Autodesk Inventor part; units mm, degrees
ref_plane "YZ Plane" through (0, 0, 0) normal (1, 0, 0) x (0, 1, 0)
ref_plane "XZ Plane" through (0, 0, 0) normal (0, 1, 0) x (-1, 0, 0)
ref_plane "XY Plane" through (0, 0, 0) normal (0, 0, 1) x (1, 0, 0)
sketch "Sketch2" plane through (0, 0, 0) normal (0, 0, 1) x (0, 1, 0)
  line L0 (24.9, -57.75) -> (24.9, -91.85)
  circle A0 centre (24.9, -74.8) radius 17.05
  circle A1 centre (24.9, -74.8) radius 0.9375
  line L1 (24.9, -74.8) -> (36.9562, -86.8562)
  line L2 (24.9, -74.8) -> (41.95, -74.8) construction
  line L3 (26.7738, -76.6738) -> (35.0823, -84.9823) construction
  line L4 (26.3319, -77.1158) -> (34.6404, -85.4243)
  line L5 (35.5243, -84.5404) -> (27.2158, -76.2319)
  arc A2 (27.2158, -76.2319) -> (26.3319, -77.1158) centre (26.7738, -76.6738) ccw
  arc A3 (34.6404, -85.4243) -> (35.5243, -84.5404) centre (35.0823, -84.9823) ccw
  line L6 (30.9281, -80.8281) -> (42.6781, -80.8281) construction
  line L7 (34.8, -54.9) -> (34.8, -60.9186) construction
  line L8 (32.3, -54.9) -> (32.3, -60.9186)
  line L9 (37.3, -60.9186) -> (37.3, -54.9)
  arc A4 (37.3, -54.9) -> (32.3, -54.9) centre (34.8, -54.9) ccw
  arc A5 (32.3, -60.9186) -> (37.3, -60.9186) centre (34.8, -60.9186) ccw
  line L10 (15, -54.9) -> (15, -60.9186) construction
  line L11 (12.5, -54.9) -> (12.5, -60.9186)
  line L12 (17.5, -60.9186) -> (17.5, -54.9)
  arc A6 (17.5, -54.9) -> (12.5, -54.9) centre (15, -54.9) ccw
  arc A7 (12.5, -60.9186) -> (17.5, -60.9186) centre (15, -60.9186) ccw
  line L13 (15, -94.7) -> (15, -88.6814) construction
  line L14 (17.5, -94.7) -> (17.5, -88.6814)
  line L15 (12.5, -88.6814) -> (12.5, -94.7)
  arc A8 (12.5, -94.7) -> (17.5, -94.7) centre (15, -94.7) ccw
  arc A9 (17.5, -88.6814) -> (12.5, -88.6814) centre (15, -88.6814) ccw
  line L16 (34.8, -94.7) -> (34.8, -88.6814) construction
  line L17 (37.3, -94.7) -> (37.3, -88.6814)
  line L18 (32.3, -88.6814) -> (32.3, -94.7)
  arc A10 (32.3, -94.7) -> (37.3, -94.7) centre (34.8, -94.7) ccw
  arc A11 (37.3, -88.6814) -> (32.3, -88.6814) centre (34.8, -88.6814) ccw
  line L19 (39.3, -74.175) -> (27.55, -74.175)
  arc A12 (39.3, -75.425) -> (39.3, -74.175) centre (39.3, -74.8) ccw
  line L20 (27.55, -75.425) -> (39.3, -75.425)
  arc A13 (27.55, -74.175) -> (27.55, -75.425) centre (27.55, -74.8) ccw
  line L21 (34.6404, -64.1757) -> (26.3319, -72.4842)
  arc A14 (35.5243, -65.0596) -> (34.6404, -64.1757) centre (35.0823, -64.6177) ccw
  line L22 (27.2158, -73.3681) -> (35.5243, -65.0596)
  arc A15 (26.3319, -72.4842) -> (27.2158, -73.3681) centre (26.7738, -72.9262) ccw
  line L23 (24.275, -60.4) -> (24.275, -72.15)
  arc A16 (25.525, -60.4) -> (24.275, -60.4) centre (24.9, -60.4) ccw
  line L24 (25.525, -72.15) -> (25.525, -60.4)
  arc A17 (24.275, -72.15) -> (25.525, -72.15) centre (24.9, -72.15) ccw
  line L25 (14.2757, -65.0596) -> (22.5842, -73.3681)
  arc A18 (15.1596, -64.1757) -> (14.2757, -65.0596) centre (14.7177, -64.6177) ccw
  line L26 (23.4681, -72.4842) -> (15.1596, -64.1757)
  arc A19 (22.5842, -73.3681) -> (23.4681, -72.4842) centre (23.0262, -72.9262) ccw
  line L27 (10.5, -75.425) -> (22.25, -75.425)
  arc A20 (10.5, -74.175) -> (10.5, -75.425) centre (10.5, -74.8) ccw
  line L28 (22.25, -74.175) -> (10.5, -74.175)
  arc A21 (22.25, -75.425) -> (22.25, -74.175) centre (22.25, -74.8) ccw
  line L29 (15.1596, -85.4243) -> (23.4681, -77.1158)
  arc A22 (14.2757, -84.5404) -> (15.1596, -85.4243) centre (14.7177, -84.9823) ccw
  line L30 (22.5842, -76.2319) -> (14.2757, -84.5404)
  arc A23 (23.4681, -77.1158) -> (22.5842, -76.2319) centre (23.0262, -76.6738) ccw
  line L31 (25.525, -89.2) -> (25.525, -77.45)
  arc A24 (24.275, -89.2) -> (25.525, -89.2) centre (24.9, -89.2) ccw
  line L32 (24.275, -77.45) -> (24.275, -89.2)
  arc A25 (25.525, -77.45) -> (24.275, -77.45) centre (24.9, -77.45) ccw
  line L33 (37.3, -60.9186) -> (37.3, -88.6814)
  line L34 (12.5, -88.6814) -> (12.5, -60.9186)
  line L35 (0.025, -97.7) -> (0.025, -51.9)
  line L36 (42.1, -97.7) -> (0.025, -97.7)
  line L37 (42.1, -97.7) -> (42.1, -91.85)
  line L38 (7.7, -91.85) -> (42.1, -91.85)
  line L39 (7.7, -57.75) -> (7.7, -91.85)
  line L40 (7.7, -57.75) -> (42.1, -57.75)
  line L41 (42.1, -57.75) -> (42.1, -51.9)
  line L42 (0.025, -51.9) -> (42.1, -51.9)
  circle A26 centre (34.8, -94.7) radius 2.0625
  circle A27 centre (34.8, -54.9) radius 2.0625
  circle A28 centre (15, -94.7) radius 2.0625
  circle A29 centre (15, -54.9) radius 2.0625
  point P0 (0, 0)
  point P1 (34.8, -57.9093)
  point P2 (15, -57.9093)
  point P3 (15, -91.6907)
  point P4 (34.8, -91.6907)
  point P5 (17.5, -59.4396)
  point P6 (13.0765, -62.5156)
  point P7 (13.0765, -87.0844)
  point P8 (17.5, -90.1604)
  point P9 (32.3, -90.1604)
  point P10 (36.7235, -87.0844)
  point P11 (36.7235, -62.5156)
  point P12 (32.3, -59.4396)
  point P13 (12.5, -63.0978)
  point P14 (12.5, -86.5022)
  point P15 (37.3, -86.5022)
  point P16 (37.3, -63.0978)
  dimension "d32" = 1.875
  dimension "d33" = 45
  dimension "d34" = 5.875
  dimension "d35" = 45
  dimension "d36" = 1.25
  dimension "d37" = 5
  dimension "d38" = 5
  dimension "d39" = 5
  dimension "d40" = 5
  dimension "d43" = 360
extrude "Extrusion2" add sketch "Sketch2" along normal mid plane 2.5 contours A0 L8 A5 L33 L19 A13 L20 L1 A3 L5 A2 A1 L0 A17 L24 A16 | L0 A16 L23 A17 A1 A25 L32 A24 A0 L14 A9 L34 L27 A21 L28 A7 L12 | L8 L40 L9 A5 A0 | A0 A5 L8 | L12 A7 A0 | A0 A7 L11 L40 L12 | L40 L11 A6 L12 | L8 A4 L9 L40 | A5 L33 A0 | A0 L34 A7 | A0 L33 L20 A12 L19 | L34 L28 A20 L27 A0 | A1 L1 A2 L4 A3 A0 A11 L18 L0 A24 L31 A25 | A0 A9 L34 | L33 A11 A0 | A9 L14 A0 | A0 L14 L38 L15 A9 | L38 L14 A8 L15 | L17 L38 L18 A0 A11 | A0 L18 A11 | L17 A10 L18 L38 | A26 | A27 | A28 | A29
sketch "Sketch3" plane through (0, 0, 1.25) normal (0, 0, 1) x (1, 0, 0)
  line L0 (97.7, 0.025) -> (51.9, 0.025)
  line L1 (97.7, 42.1) -> (97.7, 0.025)
  line L2 (97.7, 42.1) -> (91.85, 42.1)
  line L3 (91.85, 7.7) -> (91.85, 42.1)
  line L4 (57.75, 7.7) -> (91.85, 7.7)
  line L5 (57.75, 7.7) -> (57.75, 42.1)
  line L6 (57.75, 42.1) -> (51.9, 42.1)
  line L7 (51.9, 0.025) -> (51.9, 42.1)
  circle A0 centre (94.7, 34.8) radius 2.0625
  circle A1 centre (54.9, 34.8) radius 2.0625
  circle A2 centre (94.7, 15) radius 2.0625
  circle A3 centre (54.9, 15) radius 2.0625
  point P0 (0, 0)
extrude "Extrusion3" add sketch "Sketch3" along normal blind 5 contours A0 | A1 | A2 | A3
chamfer "Chamfer1" distance 5 angle 1 1 edges at (52.8375, 34.8, 6.25) measured on face at (52.8642, 35.1308, 2.9167)
chamfer "Chamfer2" distance 5 angle 2.5 1 edges at (92.6375, 34.8, 6.25) measured on face at (95.5842, 36.6634, 4.5833)
chamfer "Chamfer3" distance 5 angle 2.5 1 edges at (52.8375, 15, 6.25) measured on face at (56.9358, 14.6692, 4.5833)
chamfer "Chamfer4" distance 5 angle 2.5 1 edges at (92.6375, 15, 6.25) measured on face at (93.8158, 13.1366, 4.5833)
properties part number "Laser Alignment Tool V2"
Input: part model. Units: mm. Frame: model coordinates. A direction names the side the tool comes from. Round coordinates to 2 decimals unless told otherwise and drop trailing zeros. Loops run counter-clockwise (first coordinate to the right, second up) from the corner with the lowest first, then second, coordinate; pieces in that order, holes last. Notation, with made-up numbers: (39.25, -37) -> (45.25, -37) arc R21 cw to (45.25, -25) -> close; hole circle Ø1 at (9, 22.5). An arc over 180 degrees is marked (long way). Use one line per item in the form item = value. Start each with the question number.
Item 1: Section query C-C on x = 61.5. Return the cut outline in (y, z) (3 decimals).
Item 2: Contact query for flat-ended pins moving along their axis: pin 1 Ø2 at (y, z) = (36, 0.5) entering from -X; pin 2 Ø3 at (y, z) = (18.5, -0.5) entering from +X; pin 3 Ø3 at (x, z) = (90, 0.5) entering from -Y; pin 4 Ø4 at (x, z) = (77.5, 4.5) entering from +Y. Output: stop coordinate, or through.
Item 3: Section query D-D on z = 5.5. Return the cut outline in (x, y).
Item 4: Material intervals for L1, parallel to Y at x = 67, z = 0 (3 decimals); L2, parallel to Z at x = 61.5, y = 15; L3, parallel to X at y = 15, z = 4, sorted ascending. Write a range as from..to.
Item 5: Mould query, pull axis Y, two halves, no side actions, for faces 1 (the face through (74.98, 7.85, -0.02)), 2 (the face through (57, 17.5, 0)), 3 (the face through (69.5, 20.9, -1.25)). Classes: pulls with the +Y half, pulls with the -Y half, needs draft (parallel to the pull), parting line crosses it, or undercut.
Item 6: Set-up query: faces 4 (the face through (91, 12.5, 0)), 5 (the face through (66, 24.275, 0)), 6 (the face through (92, 17.5, 0)). Return all of +Z, -Z, +X, -X, +Y, -Y with unobstructed straight access to the full face (end or side cutting, diameter ignored); none if empty.
Item 7: Section query A-A on x = 74.8. Count the separate pieces of the cut face and the enclosed holes in it, then the cut area to 3 significant figures.
Ans:
q1.outline = (12.5, -1.25) -> (24.275, -1.25) -> (24.275, 1.25) -> (12.5, 1.25) -> close; (25.525, -1.25) -> (37.3, -1.25) -> (37.3, 1.25) -> (25.525, 1.25) -> close
q2.pin_1 = 52.41
q2.pin_2 = 96.2
q2.pin_3 = 12.5
q2.pin_4 = through
q3.outline = circle Ø3.98 at (54.9, 34.8); circle Ø3.75 at (54.9, 15); circle Ø3.75 at (94.7, 15); circle Ø3.75 at (94.7, 34.8)
q4.L1 = 9.739..16.216, 17.984..24.275, 25.525..31.816, 33.584..40.061
q4.L2 = -1.25..1.25
q4.L3 = 52.96..56.84, 92.76..96.64
q5.face_1 = pulls with the -Y half
q5.face_2 = undercut
q5.face_3 = needs draft
q6.face_4 = +Z, -Z, +X, -Y
q6.face_5 = +Z, -Z
q6.face_6 = +Z, -Z, +X
q7.separate_pieces = 4
q7.enclosed_holes = 0
q7.area = 15.6 mm^2
